Source: CAD feature listing. Evaluate the final solid. Frame: model axes, mm. Face numbers are marked on the shaded views. A direction names the side the tool comes from. Round coordinates to 2 decimals unless told otherwise and drop trailing zeros. Loops run counter-clockwise (first coordinate to the right, second up) from the corner with the lowest first, then second, coordinate; pieces in that order, holes last. Notation, with made-up numbers: M -23,70 L 3,70 A31 cw 3,95 Z; hole C -20,-16.75 d7. An arc over 180 degrees is marked long. Write each question's results on one line, items separated by ' | '. Start each with the question number.
1. Contact query for flat-ended pins moving along their axis: pin 1 Ø6 at (y, z) = (2.5, 30) entering from -X; pin 2 Ø0.9 at (x, z) = (21.5, 1.5) entering from +Y; pin 3 Ø1.5 at (x, z) = (22, 3) entering from -Y; pin 4 Ø5 at (x, z) = (19.5, 26.5) entering from +Y. Output: stop coordinate, or through.
2. Section B-B on y = -6.25. Output: boundary loops of the cut face in (x, z).
3. Set-up query: the marked faces 1, 2, 3 and 4. Return all of +Z, -Z, +X, -X, +Y, -Y with unobstructed straight access to the full face (end or side cutting, diameter ignored); none if empty.
4. Section C-C on x = 7.5. Output: boundary loops of the cut face in (y, z), and give its area (3 significant figures).
5. Section D-D on x = 16. Output: boundary loops of the cut face in (y, z).
6. Section A-A on z = 3.5. Output: boundary loops of the cut face in (x, y), and give its area (3 significant figures).
7. Ray query, line 1 (Z direction, x = -17, y = 1); line 2 (X direction, y = -0.25, z = 21); line 3 (Y direction, x = -3.5, z = 18.5). Return the intervals inside material, ascending.
from build123d import *

# Parameters (mm, degrees)
SKETCH_1_W             = 41.6
SKETCH_1_H             = 19.8
EXTRUDE_1_DEPTH        = 5
SKETCH_2_W             = 5
SKETCH_2_H             = 4.9
EXTRUDE_2_DEPTH        = 4
FILLET_1_R             = 1
FILLET_1_OF_MIRROR_1_R = 1
SKETCH_3_W             = 30
SKETCH_3_H             = 19.8
EXTRUDE_3_DEPTH        = 30
DRAFT_START            = 11.013057662
DRAFT_1_OUTLINE_W      = 30
DRAFT_1_OUTLINE_H      = 35
DRAFT_1_DEPTH          = 10.2606043
FILLET_2_R             = 3


# Read off the part's stored shape, not the designer's step: 구배1
with BuildPart() as part:
    # 스케치1 → 보스-돌출1 (new body)
    with BuildSketch(Plane.XY):
        Rectangle(SKETCH_1_W, SKETCH_1_H)
    extrude(amount=EXTRUDE_1_DEPTH)

    # 스케치2 → 보스-돌출2 (add)
    with BuildSketch(Plane(origin=(20.8, 0, 0), x_dir=(0, 0, -1), z_dir=(1, 0, 0))):
        with Locations((-2.5, 0.1)):
            Rectangle(SKETCH_2_W, SKETCH_2_H)
    extrude_2 = extrude(amount=EXTRUDE_2_DEPTH)

    # 필렛1
    fillet_1_edges = [part.edges().sort_by_distance(p)[0] for p in [
        (24.8, 2.55, 2.5),
        (24.8, -2.35, 2.5),
    ]]
    fillet(fillet_1_edges, radius=FILLET_1_R)

    # 대칭 복사1: 보스-돌출2 across plane
    add(extrude_2.mirror(Plane(origin=(0, 0, 0), x_dir=(0, 0, 1), z_dir=(1, 0, 0))))

    # 필렛1 of 대칭 복사1
    fillet_1_of_mirror_1_edges = [part.edges().sort_by_distance(p)[0] for p in [
        (-24.8, 2.55, 2.5),
        (-24.8, -2.35, 2.5),
    ]]
    fillet(fillet_1_of_mirror_1_edges, radius=FILLET_1_OF_MIRROR_1_R)

    # 스케치3 → 보스-돌출3 (add)
    with BuildSketch(Plane.XY.offset(5)):
        Rectangle(SKETCH_3_W, SKETCH_3_H)
    extrude(amount=EXTRUDE_3_DEPTH)

    # 구배1 outline → 구배1 (cut)
    with BuildSketch(Plane(origin=(0, 0, 0), x_dir=(1, 0, 0), z_dir=(0, 0.9396926207859083, 0.3420201433256691)).offset(DRAFT_START)):
        with Locations((0, -17.5)):
            Rectangle(DRAFT_1_OUTLINE_W, DRAFT_1_OUTLINE_H)
    extrude(amount=DRAFT_1_DEPTH, mode=Mode.SUBTRACT)

    # 필렛2
    fillet_2_edges = [part.edges().sort_by_distance(p)[0] for p in [
        (15, 4.440446486, 20),
        (-15, 4.440446486, 20),
        (0, -1.019107028, 35),
    ]]
    fillet(fillet_2_edges, radius=FILLET_2_R)


solid = part.part
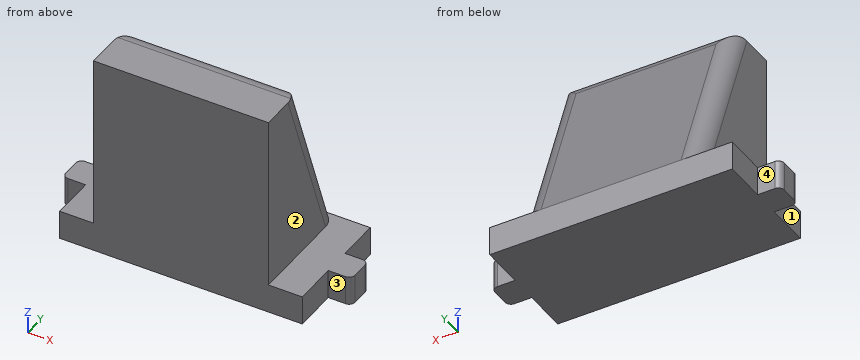
Taken from the geometry:
1) pin 1: x = -14.54 | pin 2: y = 2.55 | pin 3: y = -2.35 | pin 4: through
2) outline: M -20.8,0 L 20.8,0 L 20.8,5 L 15,5 L 15,35 L -15,35 L -15,5 L -20.8,5 Z
3) face 1: +Z, -Z, -X, -Y | face 2: +Z, +X, +Y, -Y | face 3: +Z, -Z, +X, -Y | face 4: +Z, -Z, -X, +Y
4) outline: M -9.9,0 L 9.9,0 L 9.9,5 L -0.3,33.03 A3 ccw -3.12,35 L -9.9,35 Z | area: 528 mm^2
5) outline: M -9.9,0 L 9.9,0 L 9.9,5 L -9.9,5 Z
6) outline: M -24.8,-1.35 A1 ccw -23.8,-2.35 L -20.8,-2.35 L -20.8,-9.9 L 20.8,-9.9 L 20.8,-2.35 L 23.8,-2.35 A1 ccw 24.8,-1.35 L 24.8,1.55 A1 ccw 23.8,2.55 L 20.8,2.55 L 20.8,9.9 L -20.8,9.9 L -20.8,2.55 L -23.8,2.55 A1 ccw -24.8,1.55 Z | area: 862 mm^2
7) line 1: 0 to 5 | line 2: -15 to 15 | line 3: -9.9 to 4.99
